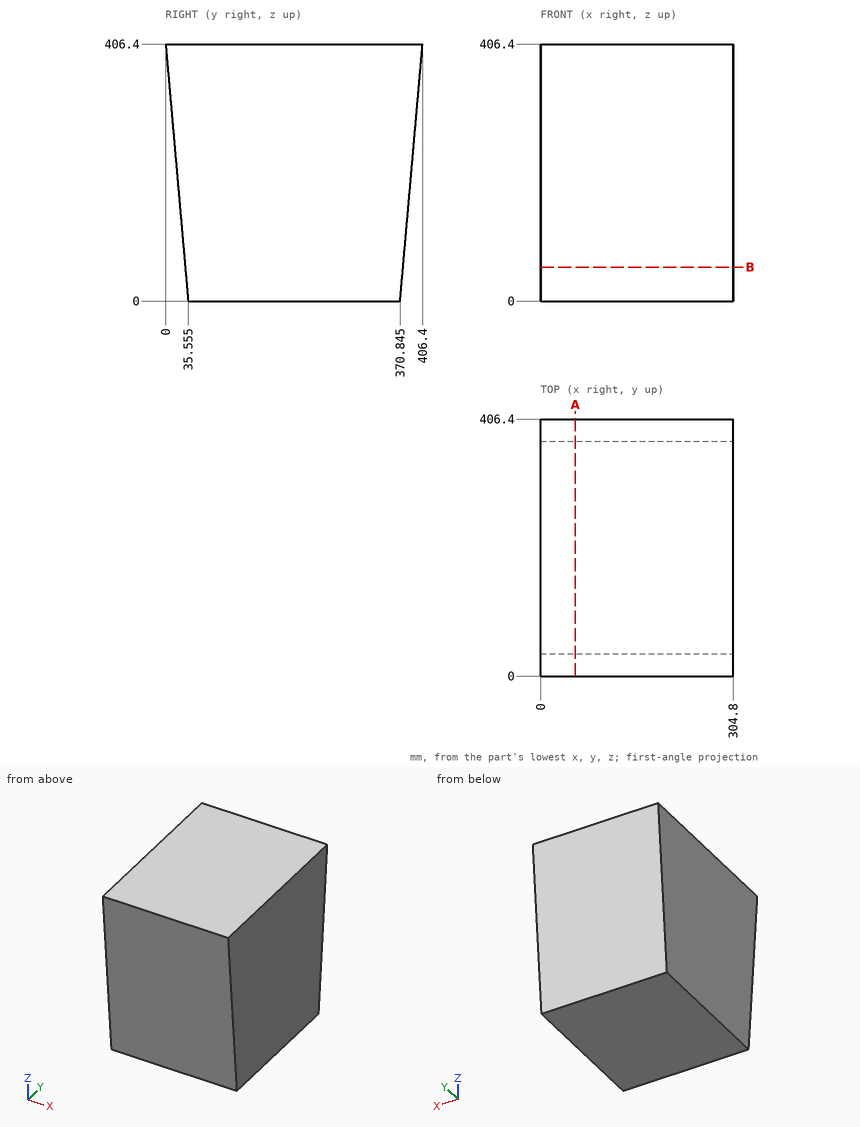
Study the drawing (mm; zero at the part's minimum x, y, z) and answer. Coordinates: 2 decimals unless noted, no trailing zeros. Order: outer loops, then holes, each group sorted by start corner. A loop starts at its lowest first (then second) coordinate and runs counter-clockwise, first axis right, second up. Notation, with made-up numbers: M -20.75,54.25 L 24.25,54.25 A13 ccw 24.25,74.25 Z; hole C 82.25,76.5 d10. An arc over 180 degrees is marked long. Answer as a JSON object with one key per item and string values. Group by question number.
1. Section B-B on z = 53.5 is taken. Write down the section's boundary in (x, y) (1 decimal), then the cut area to 3 significant figures.
2. Straight lines are drawn through the part: line 1 (Y direction, x = 181, z = 154); line 2 (Y direction, x = 241, z = 384). For each, find the intervals that lie inside material, in ascending order.
3. Section A-A on x = 55 is taken. Write down the section's boundary in (y, z) (1 decimal), then the cut area to 3 significant figures.
4. Flat-ended cylindrical pins translate along their axes: P1, Ø6, axis at x = 210.5, z = 309, coming from the +Y side; P2, Ø8, axis at x = 104.5, z = 186, coming from the +Y side; P3, Ø1, axis at x = 96, z = 78.5, coming from the -Y side. Find the tip coordinate at first contact, or state that the pin passes through.
Values follow:
{
 "1": {"outline": "M 0,30.9 L 304.8,30.9 L 304.8,375.5 L 0,375.5 Z", "area": "105,000 mm2"},
 "2": {"line 1": "22.08 to 384.32", "line 2": "1.96 to 404.44"},
 "3": {"outline": "M 0,406.4 L 35.6,0 L 370.8,0 L 406.4,406.4 Z", "area": "151,000 mm2"},
 "4": {"P1": "y = 398.14", "P2": "y = 387.47", "P3": "y = 28.64"}
}
